Autodesk Inventor part; units mm, degrees
ref_plane "YZ Plane" through (0, 0, 0) normal (1, 0, 0) x (0, 1, 0)
ref_plane "XZ Plane" through (0, 0, 0) normal (0, 1, 0) x (-1, 0, 0)
ref_plane "XY Plane" through (0, 0, 0) normal (0, 0, 1) x (1, 0, 0)
sketch "Sketch1" plane through (0, 0, 0) normal (0, 0, 1) x (1, 0, 0)
  line L0 (0, 15.0207) -> (0, -34.9793) construction
  line L1 (0, 15.0207) -> (50, 15.0207) construction
  line L2 (0, 0) -> (1, 0)
  line L3 (1, 0) -> (1, 1)
  line L4 (1, 1) -> (6.5, 1)
  line L5 (6.5, 1) -> (3, -2)
  line L6 (3, -2) -> (3, -17)
  line L7 (3, -17) -> (0, -18.7321)
  line L8 (0, -26.021) -> (0, -26.021)
  line L9 (0, 0) -> (0, -18.7321)
  dimension "d4" = 50
  dimension "d6" = 1
  dimension "d7" = 1
  dimension "d8" = 5.5
  dimension "d9" = 3
  dimension "d10" = 0
  dimension "d11" = 0
  dimension "d12" = 15
  dimension "d13" = 3
  dimension "d15" = 60
  dimension "d17" = 60
  dimension "d18" = 139.399
  dimension "d19" = 15.0207
  dimension "d20" = 41.0417
revolve "Revolution1" add sketch "Sketch1" angle 360 about axis through (0, 15.0207, 0) along (0, -1, 0)
sketch "Sketch2" plane through (0, 1, 0) normal (0, 1, 0) x (1, 0, 0)
  line L0 (-12.6442, -1) -> (7.3558, -1)
  line L1 (7.3558, -1) -> (7.3558, 1)
  line L2 (7.3558, 1) -> (-12.6442, 1)
  line L3 (-12.6442, 1) -> (-12.6442, -1)
  circle A0 centre (0, 0) radius 1
  dimension "d23" = 20
  dimension "d24" = 2
  dimension "d25" = 0
extrude "Extrusion1" cut sketch "Sketch2" against normal blind 1
properties part number "Pieza10 IG"
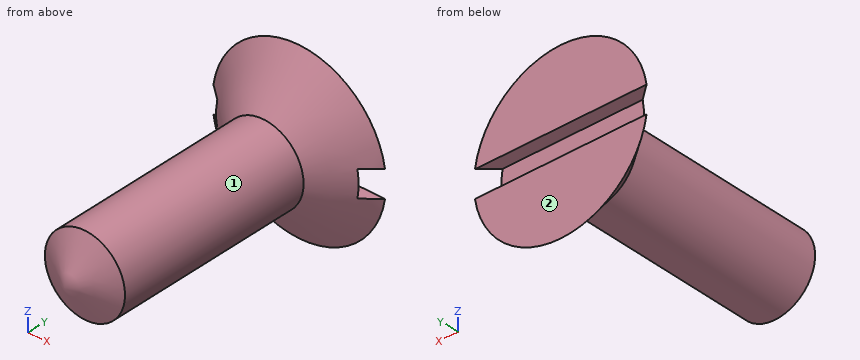
Design review of the part built by this model. Coordinates are the model's own, in mm. Face numbers are marked on the shaded views. A direction names the side the tool comes from. Give positions to 0.01 mm unless a question says otherwise; leave off trailing zeros. Write each loop counter-clockwise with the first axis right and the second up, starting at its lowest first coordinate (ties: lowest second). Pieces come first, ordered by that corner, then holes. Notation, with made-up numbers: M 36.5,6.5 L 72.5,6.5 A27 cw 72.5,38.5 Z; hole C -29,72 d4. An arc over 180 degrees is marked long. Return JSON: item names as keys, results as strings. Group by question number.
Item 1: Wall thickness on line 1 along Z through (x, y) = (4, 0.25); line 2 along Z through (x, y) = (-1.75, -3.75); line 3 along Y through (x, z) = (1, 0.5): over which ranges is each line inside the solid? List them lowest first.
Item 2: Clearance check with flat-ended pins moving along their axes: pin 1 Ø0.8 at (x, y) = (-2.5, 0.5) entering from +Z; pin 2 Ø6 at (y, z) = (-2, 1.5) entering from +X; pin 3 Ø0.5 at (x, y) = (0, 0.5) entering from -Z; pin 4 Ø2 at (y, z) = (-14.5, 5) entering from -X. State where each tip first meets the part, or that it passes through.
Item 3: Tool access review of the marked faces 1 and 2: name each direction out of +Z, -Z, +X, -X, +Y, -Y from which nothing blocks a thin tool from reaching the whole face with its end or side.
Item 4: Take a section at A-A (y = -13.5). Give the boundary of the cut face in (x, z).
Return value:
{
 "1": {"line 1": "z = -3.95 to -1, 1 to 3.95", "line 2": "z = -2.44 to 2.44", "line 3": "y = -18.09 to 0"},
 "2": {"pin 1": "stops at z = 5.9", "pin 2": "stops at x = 6.37", "pin 3": "stops at z = -6.21", "pin 4": "passes through"},
 "3": {"face 1": "-Y", "face 2": "+Z, -Z, +X, -X, +Y"},
 "4": {"outline": "C 0,0 d6"}
}
